Design review of the part shown in the three views and the two pictorial views. Dimensions are in mm from the part's minimum x, y and z. A direction names the side the tool comes from. Give positions to 0.01 mm unless a question says otherwise; leave off trailing zeros. Loops run counter-clockwise (first coordinate to the right, second up) from the corner with the lowest first, then second, coordinate; pieces in that order, holes last. Notation, with made-up numbers: (-9, 31.5) - (17, 31.5) arc R23 ccw to (17, 53.5) - close; hole circle Ø1 at (16.25, 34). An arc over 180 degrees is marked (long way). Answer in a Markdown table with one row per item.
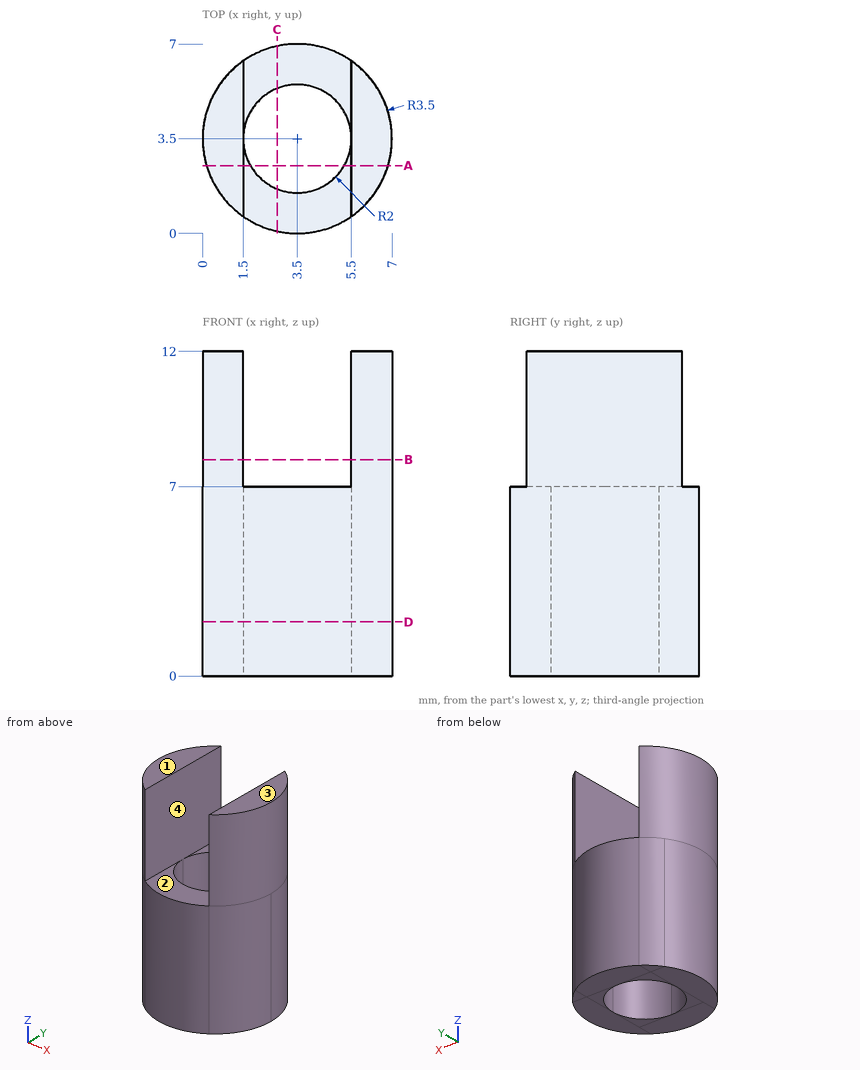
1. We need section A-A, the plane y = 2.5. Give the boundary of the cut face in (x, z), and give its area (3 significant figures).
Values:
| item | result |
|---|---|
| outline | (0.15, 0) - (1.77, 0) - (1.77, 7) - (1.5, 7) - (1.5, 12) - (0.15, 12) - close; (5.23, 0) - (6.85, 0) - (6.85, 12) - (5.5, 12) - (5.5, 7) - (5.23, 7) - close |
| area | 36.2 mm^2 |
2. Wall thickness on line 1 (X direction, y = 3.5, z = 9.25); line 2 (Z direction, x = 4, y = 5.75); line 3 (X direction, y = 2.5, z = 5.75): over which ranges is each line inside the solid? List them lowest first. Write a range as [from, to].
Values:
| item | result |
|---|---|
| line 1 | x = [0, 1.5], [5.5, 7] |
| line 2 | z = [0, 7] |
| line 3 | x = [0.15, 1.77], [5.23, 6.85] |
3. We need section B-B, the plane z = 8. Give the boundary of the cut face in (x, y).
Values:
| item | result |
|---|---|
| outline | (1.5, 0.63) - (1.5, 6.37) arc R3.5 ccw to start; (5.5, 0.63) arc R3.5 ccw to (5.5, 6.37) - close |
4. We need section D-D, the plane z = 2. Give the boundary of the cut face in (x, y), and give its area (3 significant figures).
Values:
| item | result |
|---|---|
| outline | circle Ø7 at (3.5, 3.5); hole circle Ø4 at (3.5, 3.5) |
| area | 25.9 mm^2 |
5. Mouldability with a two-part tool opening along X and no side actions: class the marked faces 1 and 2 as released by +X, released by -X, zero draft, split by the parting line, or undercut.
Values:
| item | result |
|---|---|
| face 1 | zero draft |
| face 2 | undercut |
6. We need section C-C, the plane x = 2.75. Give the boundary of the cut face in (y, z), and give its area (3 significant figures).
Values:
| item | result |
|---|---|
| outline | (0.08, 0) - (1.65, 0) - (1.65, 7) - (0.08, 7) - close; (5.35, 0) - (6.92, 0) - (6.92, 7) - (5.35, 7) - close |
| area | 21.9 mm^2 |
7. Clearance check with flat-ended pins moving along their axes: pin 1 (2.5 mm diameter, centred on y = 5, z = 10.5, fed in from +X); pin 2 (1.8 mm diameter, centred on x = 3.5, y = 2, fed in from +Z); pin 3 (2.5 mm diameter, centred on y = 5, z = 9, fed in from -X). State where each tip first meets the part, or that it passes through.
Values:
| item | result |
|---|---|
| pin 1 | stops at x = 6.99 |
| pin 2 | stops at z = 7 |
| pin 3 | stops at x = 0.01 |
8. For the marked faces 3 and 4, list the 3-axis set-ups (+Z, -Z, +X, -X, +Y, -Y) from which the entire face can be reached by the end or side of a thin tool; tool diameter is ignored.
Values:
| item | result |
|---|---|
| face 3 | +Z, +X, -X, +Y, -Y |
| face 4 | +Z, +Y, -Y |
